Drawing for the job (mm, zero at the part's lowest x, y, z). A direction names the side the tool comes from. Coordinates: 2 decimals unless noted, no trailing zeros. Order: outer loops, then holes, each group sorted by start corner. A loop starts at its lowest first (then second) coordinate and runs counter-clockwise, first axis right, second up. Notation, with made-up numbers: (-6.75, 48) - (9.25, 48) arc R24 ccw to (9.25, 64) - close; hole circle Ø2 at (-38, 40). An arc over 180 degrees is marked (long way). Answer as CSV lines item,"result". Start each with the question number.
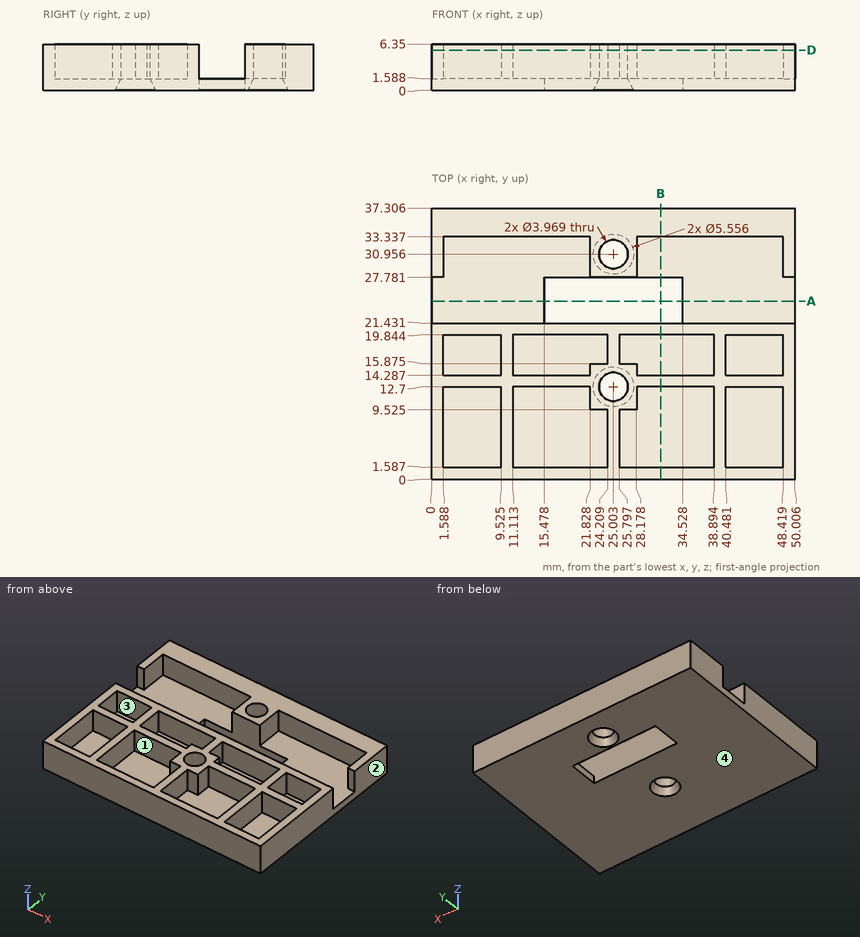
(1) Band-saw the part on A-A on y = 24.5. List the corners of the cut face in (x, z).
(2) Which spindle directions (+Z, -Z, +X, -X, +Y, -Y) get a long thin tool onto all of the face, cutting with end or side? Do the marked faces 1 and 2. Say none if no direction does.
(3) Probe L1, parallel to X at y = 28.5, z = 2.75; L2, parallel to Y at x = 7, z = 4; L3, parallel to X at y = 19, z = 2 (1 decimal). List the from-to ranges inside material, lowest first. Write a range as [from, to].
(4) Drop flat-ended pins along their axis: pin 1 Ø3 at (x, z) = (27.5, 5.5) entering from -Y; pin 2 Ø5.5 at (x, y) = (30.5, 7.5) entering from +Z. Give the stop position or say it passes through.
(5) Band-saw the part on B-B on x = 31.5. List the corners of the cut face in (y, z).
(6) Pull direction Y, two halves, no side cores. Call the marked faces 3 and 4: +Y half, -Y half, draft (parallel to the pull), parting line (faces both ways), or undercut.
(7) Band-saw the part on D-D on z = 5.5. State how many separate pieces and enclosed holes the cut face has.
Filled in:
1,outline,"(0, 0) - (15.48, 0) - (15.48, 1.59) - (0, 1.59) - close; (34.53, 0) - (50.01, 0) - (50.01, 1.59) - (34.53, 1.59) - close"
2,face 1,"+Z"
2,face 2,"+Z, -Z, +X, +Y, -Y"
3,L1,"x = [0, 1.59], [21.83, 28.18], [48.42, 50.01]"
3,L2,"y = [0, 1.59], [12.7, 14.29], [19.84, 21.43], [33.34, 37.31]"
3,L3,"x = [0, 1.6], [9.5, 11.1], [24.2, 25.8], [38.9, 40.5], [48.4, 50]"
4,pin 1,"stops at y = 0"
4,pin 2,"stops at z = 1.59"
5,outline,"(0, 0) - (21.43, 0) - (21.43, 6.35) - (19.84, 6.35) - (19.84, 1.59) - (14.29, 1.59) - (14.29, 6.35) - (12.7, 6.35) - (12.7, 1.59) - (1.59, 1.59) - (1.59, 6.35) - (0, 6.35) - close; (27.78, 0) - (37.31, 0) - (37.31, 6.35) - (33.34, 6.35) - (33.34, 1.59) - (27.78, 1.59) - close"
6,face 3,"undercut"
6,face 4,"draft"
7,separate pieces,"2"
7,enclosed holes,"10"
